from build123d import *

# Parameters (mm, degrees)
BOSS_EXTRUDE1_DEPTH = 3.5
SKETCH2_R           = 1.5
CUT_EXTRUDE1_DEPTH  = 27
SKETCH8_R           = 1.5
BOSS_EXTRUDE6_DEPTH = 1.5
SKETCH9_R           = 11
BOSS_EXTRUDE7_DEPTH = 10.5
FILLET11_R          = 3
FILLET12_R          = 3
SKETCH12_R          = 4.31867217
CUT_EXTRUDE2_DEPTH  = 1.5


with BuildPart() as part:
    # Sketch1 → Boss-Extrude1 (new, symmetric)
    with BuildSketch(Plane(origin=(0, 0, 0), x_dir=(1, 0, 0), z_dir=(0, 1, 0))):
        Polygon((-14.755737993, 80.374354469), (-9.325152651, 80.374354469), (-9.325152651, 70.474186712), (-9.539422483, 70.474186712), (-9.539422483, 55.832207765), (3.525320524, 2.274676859), (5.509138823, 2.274676859), (5.509138823, 5.883287993), (-6.679961691, 55.832207765), (-5.241843463, 55.832207765), (-5.241843463, 70.40730195), (-6.679961691, 70.40730195), (-6.679961691, 72.014475303), (-6.679961691, 80.374354469), (-5.036944489, 80.374354469), (-5.196098726, 88), (-14.755737993, 88), align=None)
    extrude(amount=BOSS_EXTRUDE1_DEPTH, both=True)

    # Sketch2 → Cut-Extrude1 (cut)
    with BuildSketch(Plane.ZY.offset(14.755737993)):
        with Locations((-85.621539819, 0)):
            Circle(SKETCH2_R)
    extrude(amount=-CUT_EXTRUDE1_DEPTH, mode=Mode.SUBTRACT)

    # Sketch8 → Boss-Extrude6 (add)
    with BuildSketch(Plane(origin=(5.509138823, 0, 0), x_dir=(0, 0, -1), z_dir=(1, 0, 0))):
        with Locations(Location((4.384839861, 0, 0), (0, 0, 2.606494438))):
            Circle(SKETCH8_R)
    extrude(amount=BOSS_EXTRUDE6_DEPTH)

    # Sketch9 → Boss-Extrude7 (add)
    with BuildSketch(Plane(origin=(7.009138823, 0, 0), x_dir=(0, 0, -1), z_dir=(1, 0, 0))):
        with Locations((4.384839861, 0)):
            Circle(SKETCH9_R)
    extrude(amount=BOSS_EXTRUDE7_DEPTH)

    # Fillet11
    fillet11_edges = [part.edges().sort_by_distance(p)[0] for p in [
        (-9.97591836, 3.5, -88),
    ]]
    fillet(fillet11_edges, radius=FILLET11_R)

    # Fillet12
    fillet12_edges = [part.edges().sort_by_distance(p)[0] for p in [
        (7.009138823, 0, 6.615160139),
        (17.509138823, 0, 6.615160139),
    ]]
    fillet(fillet12_edges, radius=FILLET12_R)

    # Sketch12 → Cut-Extrude2 (cut)
    with BuildSketch(Plane(origin=(17.509138823, 0, 0), x_dir=(0, 0, -1), z_dir=(1, 0, 0))):
        with Locations((4.384839861, 0)):
            Circle(SKETCH12_R)
    extrude(amount=-CUT_EXTRUDE2_DEPTH, mode=Mode.SUBTRACT)


solid = part.part
Input: part model. Units: mm. Frame: model coordinates. A direction names the side the tool comes from. Coordinates: 2 decimals unless noted, no trailing zeros. Loops run counter-clockwise (first coordinate to the right, second up) from the corner with the lowest first, then second, coordinate; pieces in that order, holes last. Notation, with made-up numbers: (-37.75, -3.75) -> (9.25, -3.75) arc R9 cw to (9.25, 11.25) -> close; hole circle Ø7 at (-22.5, 11). An arc over 180 degrees is marked (long way). One line per item, written item: value.
(1) Pin query (flat end, axial travel): pin 1 Ø2 at (y, z) = (-1.5, -74) entering from -X; pin 2 Ø0.7 at (x, y) = (-6, 1.5) entering from -Z; pin 3 Ø16 at (x, z) = (-5, -49) entering from +Y. Return the tip coordinate at first contact, or that it passes through.
Answer below:
pin 1: stops at x = -9.33
pin 2: stops at z = -87.93
pin 3: stops at y = 3.5
(2) Ray query, line 1 along Z through (x, y) = (-10.75, 0); line 2 along X through (y, z) = (-2.75, -80.5); line 3 along X through (y, z) = (-6.25, -3.5). Return the intervals inside material, ascending.
Answer below:
line 1: z = -88 to -87.12, -84.12 to -80.37
line 2: x = -14.76 to -5.04
line 3: x = 7.01 to 17.51
(3) Cut plane A-A (z = -62). Output: boundary loops of the cut face in (x, y), then the cut area to 3 significant figures.
Answer below:
outline: (-9.54, -3.5) -> (-5.24, -3.5) -> (-5.24, 3.5) -> (-9.54, 3.5) -> close
area: 30.1 mm2
(4) Set-up query: faces 1 (the face through (-6, 0, -80.374)), 2 (the face through (-9.325, 0, -75)), 3 (the face through (-9.539, 0, -63)), 4 (the face through (16.77, -2.63, -0.96)). Return all of +Z, -Z, +X, -X, +Y, -Y with unobstructed straight access to the full face (end or side cutting, diameter ignored); none if empty.
Answer below:
face 1: +X, +Y, -Y
face 2: -X, +Y, -Y
face 3: +Z, -X, +Y, -Y
face 4: +X
(5) Cut plane C-C (x = -3.5). Output: boundary loops of the cut face in (y, z).
Answer below:
outline: (-3.5, -42.8) -> (3.5, -42.8) -> (3.5, -31.07) -> (-3.5, -31.07) -> close
(6) Draft query along X for faces 5 (the face through (-5.242, 0, -63)), 6 (the face through (5, 0, -2.275)), 7 (the face through (7.009, 0.1, -6.1)). Return one class per face: pulls with the +X half, pulls with the -X half, needs draft (parallel to the pull), parting line crosses it, or undercut.
Answer below:
face 5: pulls with the +X half
face 6: needs draft
face 7: undercut
(7) Cut plane B-B (x = 13.5). Output: boundary loops of the cut face in (y, z), then the cut area to 3 significant figures.
Answer below:
outline: circle Ø22 at (0, -4.38)
area: 380 mm2
